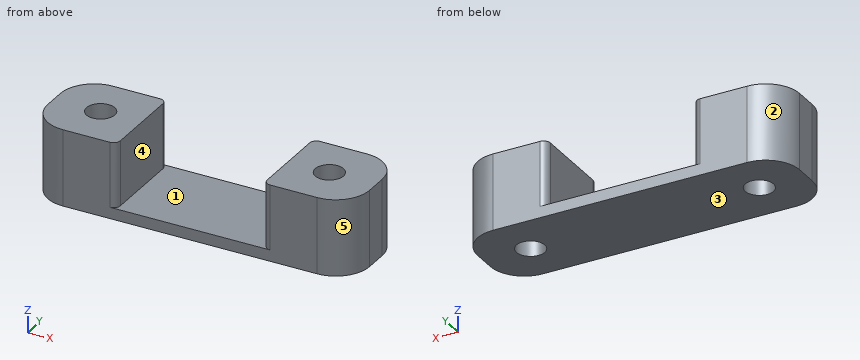
Autodesk Inventor part; units mm, degrees
ref_plane "YZ Plane" through (0, 0, 0) normal (1, 0, 0) x (0, 1, 0)
ref_plane "XZ Plane" through (0, 0, 0) normal (0, 1, 0) x (-1, 0, 0)
ref_plane "XY Plane" through (0, 0, 0) normal (0, 0, 1) x (1, 0, 0)
sketch "Sketch1" plane through (0, 0, 0) normal (0, 0, 1) x (1, 0, 0)
  line L0 (-3.0875, 5.2222) -> (9.9125, 5.2222)
  line L1 (9.9125, 5.2222) -> (9.9125, -2.7778)
  line L2 (9.9125, -2.7778) -> (-3.0875, -2.7778)
  line L3 (-3.0875, -2.7778) -> (-3.0875, 5.2222)
  line L4 (-3.0875, 5.2222) -> (-10.8375, 5.2222)
  line L5 (-10.8375, 5.2222) -> (-10.8375, -2.7778)
  line L6 (-10.8375, -2.7778) -> (-3.0875, -2.7778)
  line L7 (9.9125, -2.7778) -> (17.6625, -2.7778)
  line L8 (17.6625, -2.7778) -> (17.6625, 5.2222)
  line L9 (17.6625, 5.2222) -> (9.9125, 5.2222)
  point P0 (0, 0)
  point P1 (-6.7125, 1.2222)
  point P2 (13.5375, 1.2222)
  dimension "d0" = 13
  dimension "d1" = 8
  dimension "d2" = 7.75
  dimension "d3" = 7.75
  dimension "d6" = 4
  dimension "d7" = 4
  dimension "d22" = 20.25
  dimension "d23" = 28.5
  dimension "d24" = 4.125
extrude "Extrusion1" add sketch "Sketch1" along normal blind 5.75 contours L3 L6 L5 L4 | L9 L8 L7 L1
extrude "Extrusion2" add sketch "Sketch1" against normal blind 1
hole "Hole1" at (-6.7125, 1.2222, 0) at (13.5375, 1.2222, 0) direction (0, 0, 1) diameter 2.5 end through all both
fillet "Fillet1" radius 3 4 edges at (-10.8375, -2.7778, 2.375) (-10.8375, 5.2222, 2.375) (17.6625, -2.7778, 2.375) (17.6625, 5.2222, 2.375)
fillet "Fillet2" radius 0.6 4 edges at (9.9125, -2.7778, 2.875) (-3.0875, -2.7778, 2.875) (9.9125, 5.2222, 2.875) (-3.0875, 5.2222, 2.875)
equation "\"d3\" = d2"
properties part number "3DP_PLA_X_axis_endstop_mount" material "ABS Plastic"
Could you check a few things on this model? Use its own coordinates, in mm. Face numbers are marked on the shaded views. A direction names the side the tool comes from. Round coordinates to 2 decimals unless told otherwise and drop trailing zeros. Order: outer loops, then holes, each group sorted by start corner. A loop starts at its lowest first (then second) coordinate and runs counter-clockwise, first axis right, second up.
Q1. Imagine slicing it at B-B, the plane y = 0.75. List the corners of the cut face in (x, z) for me.
Geometry says:
outline: (-10.84, -1) - (-7.87, -1) - (-7.87, 5.75) - (-10.84, 5.75) - close; (-5.56, -1) - (12.38, -1) - (12.38, 5.75) - (9.91, 5.75) - (9.91, 0) - (-3.09, 0) - (-3.09, 5.75) - (-5.56, 5.75) - close; (14.69, -1) - (17.66, -1) - (17.66, 5.75) - (14.69, 5.75) - close
Q2. Imagine slicing it at C-C, the plane x = -6. List the corners of the cut face in (y, z) for me, then the cut area to 3 significant figures.
Geometry says:
outline: (-2.78, -1) - (0.2, -1) - (0.2, 5.75) - (-2.78, 5.75) - close; (2.25, -1) - (5.22, -1) - (5.22, 5.75) - (2.25, 5.75) - close
area: 40.1 mm2
Q3. Imagine slicing it at D-D, the plane y = 3. List the corners of the cut face in (x, z) for me.
Geometry says:
outline: (-10.73, -1) - (17.56, -1) - (17.56, 5.75) - (9.91, 5.75) - (9.91, 0) - (-3.09, 0) - (-3.09, 5.75) - (-10.73, 5.75) - close
Q4. Imagine slicing it at A-A, the plane z = 0.75. List the corners of the cut face in (x, y) for me.
Geometry says:
outline: (-10.84, 0.22) arc R3 ccw to (-7.84, -2.78) - (-3.69, -2.78) arc R0.6 ccw to (-3.09, -2.18) - (-3.09, 4.62) arc R0.6 ccw to (-3.69, 5.22) - (-7.84, 5.22) arc R3 ccw to (-10.84, 2.22) - close; (9.91, -2.18) arc R0.6 ccw to (10.51, -2.78) - (14.66, -2.78) arc R3 ccw to (17.66, 0.22) - (17.66, 2.22) arc R3 ccw to (14.66, 5.22) - (10.51, 5.22) arc R0.6 ccw to (9.91, 4.62) - close; hole circle Ø2.5 at (-6.71, 1.22); hole circle Ø2.5 at (13.54, 1.22)
Q5. I'm going to push a flat-ended pin straight in: P1, Ø3, axis at x = 13.54, y = 1.22, coming from the +Z side. Where does the tip first touch, or does it pass through?
Geometry says:
P1: stops at z = 5.75
Q6. Please list where these lines run through material, in increasing order: probe 1 along X at (y, z) = (1, 5.25); probe 2 along Z at (x, y) = (1.5, -1.25); probe 3 along X at (y, z) = (2.75, 0.5).
Geometry says:
probe 1: x = -10.84 to -7.94, -5.48 to -3.09, 9.91 to 12.31, 14.77 to 17.66
probe 2: z = -1 to 0
probe 3: x = -10.79 to -3.09, 9.91 to 17.62
Q7. Thinking about a two-plate mould opening in X: for the marked faces 1, 2 and 3, which applies, released by +X, released by -X, zero draft, split by the parting line, or undercut?
Geometry says:
face 1: undercut
face 2: released by -X
face 3: zero draft
Q8. Which directions (+Z, -Z, +X, -X, +Y, -Y) give clear straight access to the entire face, cutting with the end or side of a thin tool? Please do the marked faces 4 and 5.
Geometry says:
face 4: +Z, +Y, -Y
face 5: +Z, -Z, +X, -Y
